```python
from build123d import *

# Parameters (mm, degrees)
RESSALTO_EXTRUS_O1_DEPTH = 1.9
ESBO_O3_R                = 0.297205441
ESBO_O3_R_2              = 0.285630525
RESSALTO_EXTRUS_O2_DEPTH = 10


with BuildPart() as part:
    # Esboço2 → Ressalto-extrusão1 (new body)
    with BuildSketch(Plane.XY):
        with BuildLine():
            Line((-1.446547614, -2.55), (1.446547614, -2.55))
            ThreePointArc((1.446547614, -2.55), (2.55, -0.45), (1.446547614, 1.65))
            Line((1.446547614, 1.65), (-1.446547614, 1.65))
            ThreePointArc((-1.446547614, 1.65), (-2.55, -0.45), (-1.446547614, -2.55))
        make_face()
    extrude(amount=RESSALTO_EXTRUS_O1_DEPTH)

    # Esboço3 → Ressalto-extrusão2 (add)
    with BuildSketch(Plane.XY.offset(2.1)):
        with Locations((1.7, -0.45)):
            Circle(ESBO_O3_R)
        with Locations((-1.7, -0.45)):
            Circle(ESBO_O3_R_2)
    extrude(amount=-RESSALTO_EXTRUS_O2_DEPTH)


solid = part.part
```
The listing builds one solid part. Answer for the finished solid, in the listing's coordinates (mm). Coordinates: 2 decimals unless noted, no trailing zeros. Loops run counter-clockwise (first coordinate to the right, second up) from the corner with the lowest first, then second, coordinate; pieces in that order, holes last. Notation, with made-up numbers: (43.25, -1.75) - (66.25, -1.75) arc R24 ccw to (66.25, 15.25) - close; hole circle Ø8 at (6, 50). An arc over 180 degrees is marked (long way). Use a Markdown table: item, result. Add a question column.
1) Find the intervals of material crossed by line 1 (Z direction, x = -0.35, y = -2.35); line 2 (X direction, y = -0.35, z = -2.5); line 3 (X direction, y = -0.6, z = -7), in increasing order.
2) The part is cut by section A-A, the plane z = -6.5. Give the vertices of the cut face in (x, y), and give its area (3 significant figures).
3) Given pin 1 (2 mm diameter, centred on x = 0, y = 0, fed in from +Z); pin 2 (2 mm diameter, centred on y = -2, z = 0.5, fed in from +X); pin 3 (2 mm diameter, centred on x = -0.5, y = -1.5, fed in from -Z), each flat-ended and moving along its own axis, determine where each tip first touches the part or whether it passes through.
4) The part is cut by section C-C, the plane x = 1.7. Give the vertices of the cut face in (y, z).
5) The part is cut by section B-B, the plane y = -0.45. Give the vertices of the cut face in (x, z), and give its area (3 significant figures).
6) The part is cut by section D-D, the plane x = -1.7. Give the vertices of the cut face in (y, z).
Here are the results:
| question | item | result |
|---|---|---|
| 1 | line 1 | z = 0 to 1.9 |
| 1 | line 2 | x = -1.97 to -1.43, 1.42 to 1.98 |
| 1 | line 3 | x = -1.94 to -1.46, 1.44 to 1.96 |
| 2 | outline | circle Ø0.57 at (-1.7, -0.45); circle Ø0.59 at (1.7, -0.45) |
| 2 | area | 0.534 mm^2 |
| 3 | pin 1 | stops at z = 1.9 |
| 3 | pin 2 | stops at x = 2.49 |
| 3 | pin 3 | stops at z = 0 |
| 4 | outline | (-2.35, 0) - (-0.75, 0) - (-0.75, -7.9) - (-0.15, -7.9) - (-0.15, 0) - (1.45, 0) - (1.45, 1.9) - (-0.15, 1.9) - (-0.15, 2.1) - (-0.75, 2.1) - (-0.75, 1.9) - (-2.35, 1.9) - close |
| 5 | outline | (-2.55, 0) - (-1.99, 0) - (-1.99, -7.9) - (-1.41, -7.9) - (-1.41, 0) - (1.4, 0) - (1.4, -7.9) - (2, -7.9) - (2, 0) - (2.55, 0) - (2.55, 1.9) - (2, 1.9) - (2, 2.1) - (1.4, 2.1) - (1.4, 1.9) - (-1.41, 1.9) - (-1.41, 2.1) - (-1.99, 2.1) - (-1.99, 1.9) - (-2.55, 1.9) - close |
| 5 | area | 19.1 mm^2 |
| 6 | outline | (-2.35, 0) - (-0.74, 0) - (-0.74, -7.9) - (-0.16, -7.9) - (-0.16, 0) - (1.45, 0) - (1.45, 1.9) - (-0.16, 1.9) - (-0.16, 2.1) - (-0.74, 2.1) - (-0.74, 1.9) - (-2.35, 1.9) - close |
